Answer from the drawing. Dimensions are ordinates in mm from the lowest x, y and z of the part. Round coordinates to 2 decimals unless told otherwise and drop trailing zeros. Order: outer loops, then holes, each group sorted by start corner. A loop starts at its lowest first (then second) coordinate and runs counter-clockwise, first axis right, second up.
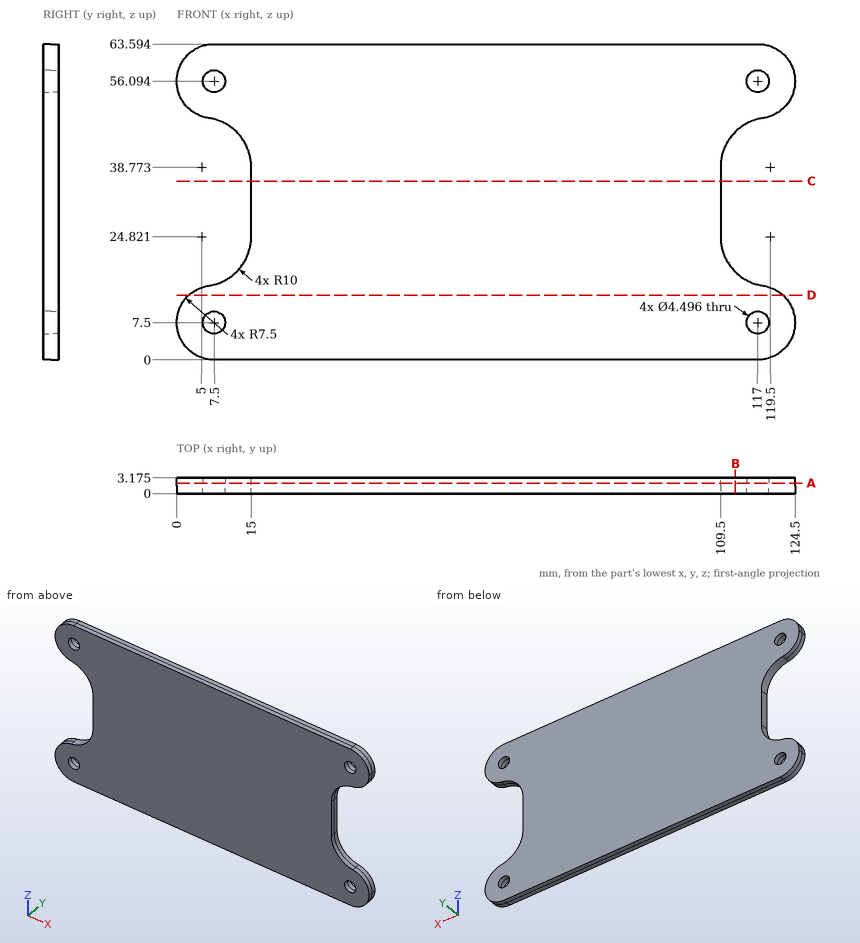
Q1. Straight lines are drawn through the part: probe 1 along X at (y, z) = (1.1, 7.5); probe 2 along X at (y, z) = (0.55, 31); probe 3 along X at (y, z) = (2.1, 19). For each, find the intervals that lie inside material, in ascending order.
Outcome:
probe 1: x = 0 to 5.25, 9.75 to 114.75, 119.25 to 124.5
probe 2: x = 15 to 109.5
probe 3: x = 13.13 to 111.37
Q2. A cutting plane is placed at A-A, the plane y = 2.1. Give the vertices of the cut face in (x, z) (1 decimal), plus the area to 3 significant figures.
Outcome:
outline: (6.4, 14.9) arc R7.5 ccw to (7.5, 0) - (117, 0) arc R7.5 ccw to (118.1, 14.9) arc R10 cw to (109.5, 24.8) - (109.5, 38.8) arc R10 cw to (118.1, 48.7) arc R7.5 ccw to (117, 63.6) - (7.5, 63.6) arc R7.5 ccw to (6.4, 48.7) arc R10 cw to (15, 38.8) - (15, 24.8) arc R10 cw to start; hole circle Ø4.5 at (7.5, 7.5); hole circle Ø4.5 at (7.5, 56.1); hole circle Ø4.5 at (117, 7.5); hole circle Ø4.5 at (117, 56.1)
area: 6,830 mm2
Q3. Flat-ended cylindrical pins translate along their axes: pin 1 (7 mm diameter, centred on x = 7.5, z = 56.094, fed in from -Y); pin 2 (1 mm diameter, centred on y = 2.5, z = 39.5, fed in from -X) (1 decimal); pin 3 (0.5 mm diameter, centred on y = 1, z = 29.5, fed in from +X). Find the tip coordinate at first contact, or state that the pin passes through.
Outcome:
pin 1: stops at y = 0
pin 2: stops at x = 14.9
pin 3: stops at x = 109.5
Q4. A cutting plane is placed at B-B, the plane x = 112.5. Give the vertices of the cut face in (y, z) (1 decimal).
Outcome:
outline: (0, 0) - (3.2, 0) - (3.2, 17.7) - (0, 17.7) - close; (0, 45.9) - (3.2, 45.9) - (3.2, 63.6) - (0, 63.6) - close
Q5. A cutting plane is placed at D-D, the plane z = 13. Give the vertices of the cut face in (x, y) (1 decimal), plus the area to 3 significant figures.
Outcome:
outline: (2.4, 0) - (122.1, 0) - (122.1, 3.2) - (2.4, 3.2) - close
area: 380 mm2
Q6. A cutting plane is placed at C-C, the plane z = 36. Give the vertices of the cut face in (x, y) (1 decimal), plus the area to 3 significant figures.
Outcome:
outline: (15, 0) - (109.5, 0) - (109.5, 3.2) - (15, 3.2) - close
area: 300 mm2
